Model file for the job. Use its own axes, mm. A direction names the side the tool comes from. Coordinates: 2 decimals unless noted, no trailing zeros. Write each loop counter-clockwise with the first axis right and the second up, starting at its lowest first coordinate (ties: lowest second). Pieces come first, ordered by that corner, then holes. Notation, with made-up numbers: M 59,-3 L 108,-3 A16 cw 108,13 Z; hole C 57.25,11 d7. An arc over 180 degrees is marked long. One line per question, with ' | ' between items. Start each with the question number.
(1) Cut at A-A (y = 1.5). Write the cut outline in (x, z).
(2) Cut at B-B (z = -11.5). Write the cut outline in (x, y).
(3) Wall check: probe 1 along X at (y, z) = (1.25, 0); probe 2 along X at (y, z) = (-4, 5); probe 3 along Z at (x, y) = (19, -2.75). Give the ranges that are in metal, low to high.
(4) Two-plate mould, pull along X, no slides. Class faces 1 (the face through (-31.1, 6.35, -0.2)), 2 (the face through (25, 0, 0)): +X half, -X half, draft (parallel to the pull), parting line (faces both ways), or undercut.
(5) Cut at D-D (z = -20). Write the cut outline in (x, y) (3 decimals).
(6) Tool access for faces 3 (the face through (25, 2, -13.906)), 4 (the face through (18.25, 3, 0)), 5 (the face through (0, -5, 25.21)), 6 (the face through (-25, -3.175, 20)): list every direction of +Z, -Z, +X, -X, +Y, -Y with a clear straight run to the whole face (end or side of a thin tool).
(7) Flat gauge pins, fed straight in: pin 1 Ø12 at (x, z) = (-6.5, -5.5) entering from +Y; pin 2 Ø3.5 at (x, z) = (24.5, -20) entering from +Y (3 decimals); pin 3 Ø1.5 at (x, y) = (-7, -4.5) entering from +Z; pin 4 Ø6 at (x, z) = (3.5, 20) entering from +Y. Where does each tip first touch, or does it go through?
from build123d import *

# Parameters (mm, degrees)
SKETCH1_W           = 12.7
SKETCH1_H           = 21.463
BOSS_EXTRUDE1_DEPTH = 6.35
BOSS_EXTRUDE2_DEPTH = 3.175
BOSS_EXTRUDE3_DEPTH = 3.175
SKETCH4_W           = 30.1498
SKETCH4_H           = 8.763
CUT_EXTRUDE1_DEPTH  = 9.779
SKETCH6_W           = 30.1498
SKETCH6_H           = 2.921
BOSS_EXTRUDE4_DEPTH = 11.303


with BuildPart() as part:
    # Sketch1 → Boss-Extrude1 (new body)
    with BuildSketch(Plane(origin=(0, 0, 0), x_dir=(1, 0, 0), z_dir=(0, 1, 0))):
        Polygon((-34.1249, 13.9065), (-34.1249, -13.9065), (-15.0749, -13.9065), (15.0749, -13.9065), (34.1249, -13.9065), (34.1249, 13.9065), (15.0749, 13.9065), (15.0749, -5.1435), (-15.0749, -5.1435), (-15.0749, 13.9065), align=None)
        with Locations((-24.5999, 0)):
            Rectangle(SKETCH1_W, SKETCH1_H, mode=Mode.SUBTRACT)
        with Locations((24.5999, 0)):
            Rectangle(SKETCH1_W, SKETCH1_H, mode=Mode.SUBTRACT)
    extrude(amount=BOSS_EXTRUDE1_DEPTH)

    # Sketch2 → Boss-Extrude2 (add)
    with BuildSketch(Plane.XZ):
        Polygon((-15.0749, 5.1435), (-15.0749, -13.9065), (-34.1249, -13.9065), (-34.1249, 13.9065), (34.1249, 13.9065), (34.1249, -13.9065), (15.0749, -13.9065), (15.0749, 5.1435), align=None)
    extrude(amount=BOSS_EXTRUDE2_DEPTH)

    # Sketch3 → Boss-Extrude3 (add)
    with BuildSketch(Plane.XZ.offset(3.175)):
        Polygon((-34.1249, -25.4), (-15.0749, -25.4), (-15.0749, 5.1435), (15.0749, 5.1435), (15.0749, -25.4), (34.1249, -25.4), (34.1249, 25.4), (15.0749, 25.4), (15.0749, 13.9065), (-15.0749, 13.9065), (-15.0749, 25.4), (-34.1249, 25.4), align=None)
    extrude(amount=BOSS_EXTRUDE3_DEPTH)

    # Sketch4 → Cut-Extrude1 (cut)
    with BuildSketch(Plane(origin=(0, 6.35, 0), x_dir=(1, 0, 0), z_dir=(0, 1, 0))):
        with Locations((0, -9.525)):
            Rectangle(SKETCH4_W, SKETCH4_H)
    extrude(amount=-CUT_EXTRUDE1_DEPTH, mode=Mode.SUBTRACT)

    # Sketch6 → Boss-Extrude4 (add)
    with BuildSketch(Plane.XY.offset(13.9065)):
        with Locations((0, -4.8895)):
            Rectangle(SKETCH6_W, SKETCH6_H)
    extrude(amount=BOSS_EXTRUDE4_DEPTH)


solid = part.part
Filled in:
1) outline: M -34.12,-13.91 L -15.07,-13.91 L -15.07,13.91 L -34.12,13.91 Z; M 15.07,-13.91 L 34.12,-13.91 L 34.12,13.91 L 15.07,13.91 Z; hole M -30.95,-10.73 L -18.25,-10.73 L -18.25,10.73 L -30.95,10.73 Z; hole M 18.25,-10.73 L 30.95,-10.73 L 30.95,10.73 L 18.25,10.73 Z
2) outline: M -34.12,-6.35 L -15.07,-6.35 L -15.07,6.35 L -34.12,6.35 Z; M 15.07,-6.35 L 34.12,-6.35 L 34.12,6.35 L 15.07,6.35 Z
3) probe 1: -34.12 to -30.95, -18.25 to -15.07, 15.07 to 18.25, 30.95 to 34.12 | probe 2: -34.12 to -15.07, 15.07 to 34.12 | probe 3: -13.91 to 13.91
4) face 1: draft | face 2: undercut
5) outline: M -34.125,-6.35 L -15.075,-6.35 L -15.075,-3.175 L -34.125,-3.175 Z; M 15.075,-6.35 L 34.125,-6.35 L 34.125,-3.175 L 15.075,-3.175 Z
6) face 3: -Z, +X, -X, +Y | face 4: +Y | face 5: +Z, +Y, -Y | face 6: +Z, +X, -X, +Y
7) pin 1: through | pin 2: y = -3.175 | pin 3: z = 25.21 | pin 4: y = -3.43
